Model file for the job. Use its own axes, mm. A direction names the side the tool comes from. Coordinates: 2 decimals unless noted, no trailing zeros. Order: outer loops, then holes, each group sorted by start corner. A loop starts at its lowest first (then second) coordinate and runs counter-clockwise, first axis right, second up. Notation, with made-up numbers: M -20,68 L 1,68 A19 cw 1,78 Z; hole C -14.75,-7 d4. An arc over 180 degrees is marked long. Return JSON: item names as keys, results as strings.
```python
from build123d import *

# Parameters (mm, degrees)
EXTRUDE_1_DEPTH     = 5
SKETCH_2_W          = 20
SKETCH_2_H          = 3
SKETCH_2_W_2        = 10
SKETCH_2_H_2        = 30
SKETCH_2_H_3        = 50
CUT_EXTRUDE_1_DEPTH = 211.35683968
EXTRUDE_2_DEPTH     = 5
SKETCH_4_R          = 2
CUT_EXTRUDE_2_DEPTH = 620.212910153
SKETCH_6_W          = 3
SKETCH_6_H          = 50
SKETCH_6_H_2        = 104
EXTRUDE_3_DEPTH     = 5
EXTRUDE_4_DEPTH     = 5
SKETCH_8_R          = 2
SKETCH_8_W          = 50
SKETCH_8_H          = 10
CUT_EXTRUDE_3_DEPTH = 620.212910153
SKETCH_9_R          = 2
CUT_EXTRUDE_4_DEPTH = 620.212910153
SKETCH_10_R         = 7.5
CUT_EXTRUDE_5_DEPTH = 620.212910153


with BuildPart() as part:
    # 스케치1 → 보스-돌출1 (new body)
    with BuildSketch(Plane(origin=(0, 0, 0), x_dir=(1, 0, 0), z_dir=(0, 1, 0))):
        Polygon((-50, 175), (0, 175), (0, 185), (50, 185), (50, 175), (100, 175), (100, -175), (50, -175), (50, -185), (0, -185), (0, -175), (-50, -175), (-50, -185), (-100, -185), (-100, -175), (-100, 175), (-100, 185), (-50, 185), align=None)
    extrude(amount=EXTRUDE_1_DEPTH)

    # 스케치2 → 컷-돌출1 (cut, through all)
    with BuildSketch(Plane(origin=(0, 5, 0), x_dir=(1, 0, 0), z_dir=(0, 1, 0))):
        with Locations((70, 153.5)):
            Rectangle(SKETCH_2_W, SKETCH_2_H)
        with Locations((70, -153.5)):
            Rectangle(SKETCH_2_W, SKETCH_2_H)
        with Locations((45, 120)):
            Rectangle(SKETCH_2_W_2, SKETCH_2_H_2)
        with Locations((45, -120)):
            Rectangle(SKETCH_2_W_2, SKETCH_2_H_2)
        with Locations((45, 0)):
            Rectangle(SKETCH_2_W_2, SKETCH_2_H_3)
    extrude(amount=-CUT_EXTRUDE_1_DEPTH, mode=Mode.SUBTRACT)

    # 스케치3 → 보스-돌출2 (add)
    with BuildSketch(Plane(origin=(0, 5, 0), x_dir=(1, 0, 0), z_dir=(0, 1, 0))):
        Polygon((-540.91, 50), (-225, 50), (-100, 50), (-100, -50), (-225, -50), (-540.91, -50), (-540.91, -185), (-590.91, -185), (-590.91, 185), (-540.91, 185), align=None)
    extrude(amount=-EXTRUDE_2_DEPTH)

    # 스케치4 → 컷-돌출2 (cut, through all)
    with BuildSketch(Plane(origin=(0, 5, 0), x_dir=(1, 0, 0), z_dir=(0, 1, 0))):
        with Locations(Location((-578.91, 145, 0), (0, 0, 270))):
            Circle(SKETCH_4_R)
        with Locations(Location((-578.91, 95, 0), (0, 0, 270))):
            Circle(SKETCH_4_R)
        with Locations(Location((-566.91, 145, 0), (0, 0, 270))):
            Circle(SKETCH_4_R)
        with Locations(Location((-566.91, 95, 0), (0, 0, 270))):
            Circle(SKETCH_4_R)
        with Locations(Location((-578.91, -145, 0), (0, 0, 270))):
            Circle(SKETCH_4_R)
        with Locations(Location((-578.91, -95, 0), (0, 0, 270))):
            Circle(SKETCH_4_R)
        with Locations(Location((-566.91, -95, 0), (0, 0, 270))):
            Circle(SKETCH_4_R)
        with Locations(Location((-566.91, -145, 0), (0, 0, 270))):
            Circle(SKETCH_4_R)
    extrude(amount=-CUT_EXTRUDE_2_DEPTH, mode=Mode.SUBTRACT)

    # 스케치6 → 보스-돌출3 (add)
    with BuildSketch(Plane(origin=(0, 5, 0), x_dir=(1, 0, 0), z_dir=(0, 1, 0))):
        with Locations((101.5, -127)):
            Rectangle(SKETCH_6_W, SKETCH_6_H)
        with Locations((101.5, 127)):
            Rectangle(SKETCH_6_W, SKETCH_6_H)
        with Locations((101.5, 0)):
            Rectangle(SKETCH_6_W, SKETCH_6_H_2)
    extrude(amount=-EXTRUDE_3_DEPTH)

    # 스케치7 → 보스-돌출4 (add)
    with BuildSketch(Plane(origin=(0, 5, 0), x_dir=(1, 0, 0), z_dir=(0, 1, 0))):
        Polygon((-540.91, -185), (-537.91, -185), (-537.91, -92), (-495.91, -50), (-540.91, -50), align=None)
        Polygon((-537.91, 92), (-495.91, 50), (-540.91, 50), (-540.91, 185), (-537.91, 185), align=None)
        Polygon((-100, 95), (-145, 50), (-100, 50), align=None)
        Polygon((-100, -95), (-145, -50), (-100, -50), align=None)
    extrude(amount=-EXTRUDE_4_DEPTH)

    # 스케치8 → 컷-돌출3 (cut, through all)
    with BuildSketch(Plane(origin=(0, 5, 0), x_dir=(1, 0, 0), z_dir=(0, 1, 0))):
        with Locations(Location((-52, 86, 0), (0, 0, 270))):
            Circle(SKETCH_8_R)
        with Locations(Location((-52, 64, 0), (0, 0, 270))):
            Circle(SKETCH_8_R)
        with Locations(Location((26, 86, 0), (0, 0, 270))):
            Circle(SKETCH_8_R)
        with Locations(Location((26, 64, 0), (0, 0, 270))):
            Circle(SKETCH_8_R)
        with Locations(Location((-52, -86, 0), (0, 0, 90))):
            Circle(SKETCH_8_R)
        with Locations(Location((-52, -64, 0), (0, 0, 90))):
            Circle(SKETCH_8_R)
        with Locations(Location((26, -64, 0), (0, 0, 90))):
            Circle(SKETCH_8_R)
        with Locations(Location((26, -86, 0), (0, 0, 90))):
            Circle(SKETCH_8_R)
        with Locations((-13, 75)):
            Rectangle(SKETCH_8_W, SKETCH_8_H)
        with Locations((-13, -75)):
            Rectangle(SKETCH_8_W, SKETCH_8_H)
    extrude(amount=-CUT_EXTRUDE_3_DEPTH, mode=Mode.SUBTRACT)

    # 스케치9 → 컷-돌출4 (cut, through all)
    with BuildSketch(Plane(origin=(0, 5, 0), x_dir=(1, 0, 0), z_dir=(0, 1, 0))):
        with Locations(Location((-437.91, 30, 0), (0, 0, 270))):
            Circle(SKETCH_9_R)
        with Locations(Location((-235.58, 30, 0), (0, 0, 270))):
            Circle(SKETCH_9_R)
        with Locations(Location((-185.58, 30, 0), (0, 0, 270))):
            Circle(SKETCH_9_R)
        with Locations(Location((-185.58, -30, 0), (0, 0, 90))):
            Circle(SKETCH_9_R)
        with Locations(Location((-235.58, -30, 0), (0, 0, 90))):
            Circle(SKETCH_9_R)
        with Locations(Location((-437.91, -30, 0), (0, 0, 90))):
            Circle(SKETCH_9_R)
    extrude(amount=-CUT_EXTRUDE_4_DEPTH, mode=Mode.SUBTRACT)

    # 스케치10 → 컷-돌출5 (cut, through all)
    with BuildSketch(Plane(origin=(0, 5, 0), x_dir=(1, 0, 0), z_dir=(0, 1, 0))):
        with Locations(Location((-73, 0, 0), (0, 0, 270))):
            Circle(SKETCH_10_R)
    extrude(amount=-CUT_EXTRUDE_5_DEPTH, mode=Mode.SUBTRACT)


solid = part.part
```
Item 1: Pull direction X, two halves, no side cores. Call faces 4 (the flat face through (-172, 5, -3)), 5 (the flat face through (-122, 3, 73)): +X half, -X half, draft (parallel to the pull), parting line (faces both ways), or undercut.
Check result:
{"face 4": "draft", "face 5": "undercut"}
Item 2: Wall check: line 1 (X direction, y = 3.25, z = -145); line 2 (Z direction, x = 73.5, y = 1.2); line 3 (X direction, y = 2.95, z = 30). Give the ranges that are in metal, low to high.
Check result:
{"line 1": "x = -590.91 to -580.91, -576.91 to -568.91, -564.91 to -537.91, -100 to 103", "line 2": "z = -175 to -155, -152 to 152, 155 to 175", "line 3": "x = -590.91 to -439.91, -435.91 to -237.58, -233.58 to -187.58, -183.58 to 103"}
Item 3: Saw through at A-A (x = -14). Write the cut outline in (y, z).
Check result:
{"outline": "M 0,-175 L 5,-175 L 5,-80 L 0,-80 Z; M 0,-70 L 5,-70 L 5,70 L 0,70 Z; M 0,80 L 5,80 L 5,175 L 0,175 Z"}
Item 4: Saw through at B-B (z = 115). Write the cut outline in (x, y).
Check result:
{"outline": "M -590.91,0 L -537.91,0 L -537.91,5 L -590.91,5 Z; M -100,0 L 40,0 L 40,5 L -100,5 Z; M 50,0 L 103,0 L 103,5 L 50,5 Z"}
Item 5: Drop flat-ended pins along their axis: pin 1 Ø1.5 at (y, z) = (3.5, 180) entering from +X; pin 2 Ø6 at (x, z) = (-408.5, 41) entering from -Y. Give the stop position or say it passes through.
Check result:
{"pin 1": "stops at x = 50", "pin 2": "stops at y = 0"}
Item 6: 3-axis set-ups, long thin cutter, end or side, ignore diameter. For faces 1 (the flat face through (-517.2, 2.54, 71.29)), 2 (the flat face through (-172, 0, -3)), 3 (the flat face through (-517.2, 2.54, -71.29)): which of +Z, -Z, +X, -X, +Y, -Y reach the whole face in a straight line?
Check result:
{"face 1": "+Z, +Y, -Y", "face 2": "+Z, -Z, +X, -X, -Y", "face 3": "-Z, +Y, -Y"}
Item 7: Saw through at C-C (y = 3.15). Count the separate pieces of the cut face and the enclosed holes in it, and give its area (3 significant figures).
Check result:
{"separate pieces": "1", "enclosed holes": "30", "area": "137,000 mm2"}
Item 8: Saw through at D-D (x = -327.5). Write the cut outline in (y, z).
Check result:
{"outline": "M 0,-50 L 5,-50 L 5,50 L 0,50 Z"}
